Here's how the part is built. I have some questions about the finished solid (model axes, mm). Round coordinates to 2 decimals unless told otherwise and drop trailing zeros. Loops run counter-clockwise (first coordinate to the right, second up) from the corner with the lowest first, then second, coordinate; pieces in that order, holes last. Notation, with made-up numbers: M 68,-16.5 L 93,-16.5 A18 cw 93,-12.5 Z; hole C -15.5,48.25 d7. An arc over 180 degrees is marked long. Answer as a JSON object with one key per item and string values.
from build123d import *

# Parameters (mm, degrees)
SKETCH1_W           = 1.5875
SKETCH1_H           = 7.1628
BOSS_EXTRUDE1_DEPTH = 1.5875


with BuildPart() as part:
    # Sketch1 → Boss-Extrude1 (new body)
    with BuildSketch(Plane.XY):
        with BuildLine():
            ThreePointArc((-20.722796249, 4.589876297), (-23.715296357, 7.4e-08), (-20.722796383, -4.589876237))
            add(Edge.make_bspline(
                [(-20.722796383, -4.589876237), (-1.820130831, -12.924202126), (19.352380946, -5.14103201)],
                knots=[3.758177337, 3.758177337, 3.758177337, 5.578637888, 5.578637888, 5.578637888], degree=2, weights=[1, 0.61356393, 1]))
            ThreePointArc((19.352380946, -5.14103201), (22.939895377, 0), (19.352380946, 5.14103201))
            add(Edge.make_bspline(
                [(19.352380946, 5.14103201), (-1.82013063, 12.924202052), (-20.722796249, 4.589876297)],
                knots=[0.704547419, 0.704547419, 0.704547419, 2.525007961, 2.525007961, 2.525007961], degree=2, weights=[1, 0.613563933, 1]))
        make_face()
        with Locations((-18.699085792, 0)):
            Rectangle(SKETCH1_W, SKETCH1_H, mode=Mode.SUBTRACT)
        with Locations((3.632105004, 0)):
            Rectangle(SKETCH1_W, SKETCH1_H, mode=Mode.SUBTRACT)
        with Locations((-10.258658934, 0)):
            Rectangle(SKETCH1_W, SKETCH1_H, mode=Mode.SUBTRACT)
        with Locations((17.4625, 0)):
            Rectangle(SKETCH1_W, SKETCH1_H, mode=Mode.SUBTRACT)
    extrude(amount=BOSS_EXTRUDE1_DEPTH)


solid = part.part
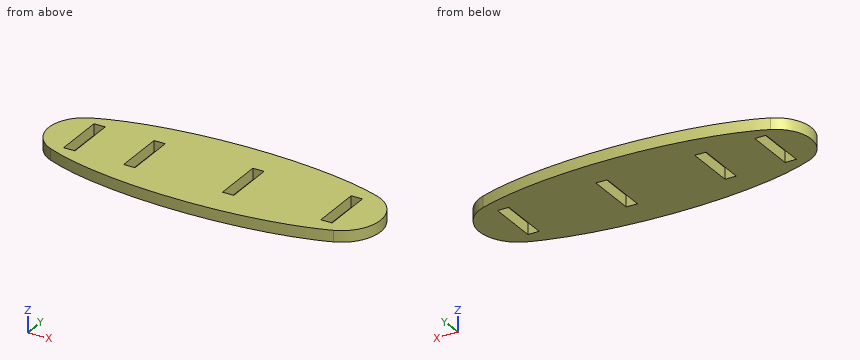
Item 1: I want a section at B-B on z = 0.7. Count the separate pieces of the cut face and the enclosed holes in it, plus the area to 3 significant figures.
Solution:
{"separate pieces": "1", "enclosed holes": "4", "area": "563 mm2"}
Item 2: I want a section at C-C on y = -4. List the corners of the cut face in (x, z) for me.
Solution:
{"outline": "M -21.73,0 L 21.2,0 L 21.2,1.59 L -21.73,1.59 Z"}
Item 3: If I drill on L1, parallel to X at y = -1.25, z = 0.7; L2, parallel to X at y = 3, z = 0.3; L3, parallel to Y at x = -11, z = 1, over which ranges is the centre line in solid material (lowest first)? Write a range as from..to.
Solution:
{"L1": "x = -23.56..-19.49, -17.91..-11.05, -9.46..2.84, 4.43..16.67, 18.26..22.8", "L2": "x = -22.72..-19.49, -17.91..-11.05, -9.46..2.84, 4.43..16.67, 18.26..22.05", "L3": "y = -7.15..-3.58, 3.58..7.15"}
Item 4: I want a section at A-A on y = -0.5. List the corners of the cut face in (x, z) for me, plus the area to 3 significant figures.
Solution:
{"outline": "M -23.69,0 L -19.49,0 L -19.49,1.59 L -23.69,1.59 Z; M -17.91,0 L -11.05,0 L -11.05,1.59 L -17.91,1.59 Z; M -9.46,0 L 2.84,0 L 2.84,1.59 L -9.46,1.59 Z; M 4.43,0 L 16.67,0 L 16.67,1.59 L 4.43,1.59 Z; M 18.26,0 L 22.92,0 L 22.92,1.59 L 18.26,1.59 Z", "area": "63.9 mm2"}
Item 5: For P1, Ø0.8, axis at x = 17.5, z = 1, coming from the -Y side; P2, Ø0.5, axis at x = 3.5, z = 1, coming from the -Y side; P3, Ø0.8, axis at y = 1.5, z = 0.5, coming from the +X side, each with a flat end and sliding along its axis, tell me the tip position at first contact or that it passes through.
Solution:
{"P1": "stops at y = -5.87", "P2": "stops at y = -7.87", "P3": "stops at x = 22.83"}
